Work out the finished part from the listing and answer in its coordinate system (mm). A direction names the side the tool comes from. Coordinates: 2 decimals unless noted, no trailing zeros. Order: outer loops, then holes, each group sorted by start corner. A loop starts at its lowest first (then second) coordinate and runs counter-clockwise, first axis right, second up.
1. Flat-ended cylindrical pins translate along their axes: pin 1 Ø6.5 at (x, z) = (6, 14) entering from +Y; pin 2 Ø6 at (x, y) = (-56.5, -6.5) entering from -Z; pin 3 Ø1.5 at (x, z) = (-53.5, -13.5) entering from -Y. Find the tip coordinate at first contact, or state that the pin passes through.
2. The part is cut by section A-A, the plane y = -9.75. Give the vertices of the cut face in (x, z).
3. The part is cut by section B-B, the plane x = -28. Give the vertices of the cut face in (y, z).
4. The part is cut by section C-C, the plane z = -0.5. Give the vertices of the cut face in (x, y).
5. A tool of negligible diameter and unlimited length cuts with its end or side. For faces 4 (the cylindrical face through (-72.49, -2.3, 19.54)), 5 (the flat face through (10, -2.5, -14)), 6 (the cylindrical face through (-35.5, 1.5, -9.23)), from which of +Z, -Z, +X, -X, +Y, -Y can it reach the whole face along a straight path? Write none if from no direction.
6. Determine the mould class of faces 1 (the flat face through (6, 0, 31)), 2 (the cylindrical face through (6, -8, 23)), 3 (the flat face through (6, 0, -31)) for opening direction Z: +Z half, -Z half, draft (parallel to the pull), parting line (faces both ways), or undercut.
7. Find the intervals of material crossed by probe 1 along Z at (x, y) = (6, -7.55); probe 2 along Z at (x, y) = (6, 8.4); probe 3 along Y at (x, z) = (7.75, -14), in increasing order.
```python
from build123d import *

# Parameters (mm, degrees)
PLATE_SKETCH_W               = 62
PLATE_SKETCH_H               = 23
PLATE_DEPTH                  = 12
TAPPED_HOLE_FACE_D           = 5
TAPPED_HOLE_FACE_CSINK_D     = 5.6
TAPPED_HOLE_FACE_CSINK_ANGLE = 90
RODS_DEPTH                   = 60
RODS_DEPTH_BACK              = 24
RODS_SKETCH_R                = 5
PISTON_SKETCH_R              = 6
PISTON_DEPTH                 = 1
TAPPED_HOLES_TOP_AT_2_COUNT  = 2
TAPPED_HOLES_TOP_AT_2_PITCH  = 50
SHCS_SEAT_SKETCH_R           = 5.5
SHCS_SEAT_DEPTH              = 6.5
SHCS_HEAD_SKETCH_R           = 5
SHCS_HEAD_DEPTH              = 6
SHCS_HEX_DEPTH               = 3
SHCS_CHAM_SIZE               = 0.6
SS_SEAT_SKETCH_R             = 4
SS_SEAT_DEPTH                = 2
SS_HEX_DEPTH                 = 4


with BuildPart() as part:
    # Plate_Sketch → Plate (new body)
    with BuildSketch(Plane(origin=(0, 0, 0), x_dir=(0, 0, -1), z_dir=(1, 0, 0))):
        Rectangle(PLATE_SKETCH_W, PLATE_SKETCH_H)
    extrude(amount=PLATE_DEPTH)

    # Tapped Hole Face (through all)
    with Locations(Plane(origin=(12, 0, 0), x_dir=(0, 0, -1), z_dir=(1, 0, 0))):
        with Locations((-25, 0), (25, 0)):
            CounterSinkHole(TAPPED_HOLE_FACE_D / 2, TAPPED_HOLE_FACE_CSINK_D / 2, counter_sink_angle=TAPPED_HOLE_FACE_CSINK_ANGLE)

    # Rods_Sketch → Rods (add, two sides: drawn at the far end of the back side and taken through both)
    with BuildSketch(Plane.ZY.offset(12).offset(-RODS_DEPTH_BACK)):
        with Locations((-14, 0)):
            Circle(RODS_SKETCH_R)
        with Locations(Location((14, 0, 0), (0, 0, 180))):
            Circle(RODS_SKETCH_R)
    extrude(amount=RODS_DEPTH + RODS_DEPTH_BACK)

    # Piston_Sketch → Piston (add)
    with BuildSketch(Plane.ZY.offset(72)):
        with Locations((-14, 0)):
            Circle(PISTON_SKETCH_R)
        with Locations((14, 0)):
            Circle(PISTON_SKETCH_R)
    extrude(amount=PISTON_DEPTH)

    # Tapped Holes Top Profile → Tapped Holes Top (revolve, cut)
    with BuildSketch(Plane(origin=(6, 11.5, -25), x_dir=(0, 0, 1), z_dir=(1, 0, 0))):
        Polygon((0, 0), (0, 6.499755867), (1.7, 6.2), (1.7, 6), (2, 6), (2, 0.3), (2.3, 0), align=None)
    tapped_holes_top = revolve(axis=Axis((6, 17.85, -25), (0, -1, 0)), mode=Mode.SUBTRACT)

    # Tapped Holes Top at 2: Tapped Holes Top ×2
    with Locations(*[(0, 0, i * TAPPED_HOLES_TOP_AT_2_PITCH) for i in range(1, TAPPED_HOLES_TOP_AT_2_COUNT)]):
        add(tapped_holes_top, mode=Mode.SUBTRACT)

    # Tapped Holes Top Mirror: Tapped Holes Top across plane
    add(tapped_holes_top.mirror(Plane.ZX), mode=Mode.SUBTRACT)

    # Tapped Holes Top Mirror copy 1 sketch → Tapped Holes Top Mirror copy 1 (revolve, cut)
    with BuildSketch(Plane(origin=(6, -11.5, 25), x_dir=(0, 0, 1), z_dir=(1, 0, 0))):
        Polygon((0, 0), (0, -6.499755867), (1.7, -6.2), (1.7, -6), (2, -6), (2, -0.3), (2.3, 0), align=None)
    revolve(axis=Axis((6, -17.85, 25), (0, -1, 0)), mode=Mode.SUBTRACT)

    # SHCS Seat_Sketch → SHCS Seat (cut)
    with BuildSketch(Plane(origin=(12, 0, 0), x_dir=(0, 0, -1), z_dir=(1, 0, 0))):
        with Locations((14, 0)):
            Circle(SHCS_SEAT_SKETCH_R)
    extrude(amount=-SHCS_SEAT_DEPTH, mode=Mode.SUBTRACT)

    # SHCS Head_Sketch → SHCS Head (add)
    with BuildSketch(Plane(origin=(5.5, 0, 0), x_dir=(0, 0, -1), z_dir=(1, 0, 0))):
        with Locations(Location((14, 0, 0), (0, 0, 180))):
            Circle(SHCS_HEAD_SKETCH_R)
    extrude(amount=SHCS_HEAD_DEPTH)

    # SHCS Hex_Sketch → SHCS Hex (cut)
    with BuildSketch(Plane(origin=(11.5, 0, 0), x_dir=(0, 0, -1), z_dir=(1, 0, 0))):
        Polygon((15.443375673, -2.5), (16.886751346, 0), (15.443375673, 2.5), (12.556624327, 2.5), (11.113248654, 0), (12.556624327, -2.5), align=None)
    extrude(amount=-SHCS_HEX_DEPTH, mode=Mode.SUBTRACT)

    # SHCS Cham
    shcs_cham_edges = [part.edges().sort_by_distance(p)[0] for p in [
        (11.5, 0, -19),
    ]]
    chamfer(shcs_cham_edges, length=SHCS_CHAM_SIZE)

    # SS Seat_Sketch → SS Seat (cut)
    with BuildSketch(Plane(origin=(0, 11.5, 0), x_dir=(-1, 0, 0), z_dir=(0, 1, 0))):
        with Locations(Location((-6, 14, 0), (0, 0, 90))):
            Circle(SS_SEAT_SKETCH_R)
    extrude(amount=-SS_SEAT_DEPTH, mode=Mode.SUBTRACT)

    # SS Hex_Sketch → SS Hex (cut)
    with BuildSketch(Plane(origin=(0, 9.5, 0), x_dir=(-1, 0, 0), z_dir=(0, 1, 0))):
        Polygon((-8, 12.845299462), (-6, 11.690598923), (-4, 12.845299462), (-4, 15.154700538), (-6, 16.309401077), (-8, 15.154700538), align=None)
    extrude(amount=-SS_HEX_DEPTH, mode=Mode.SUBTRACT)


solid = part.part
```
Geometry says:
1. pin 1: stops at y = 9.5
1. pin 2: stops at z = -17.57
1. pin 3: stops at y = -5
2. outline: (0, -31) - (12, -31) - (12, 31) - (0, 31) - close; hole circle Ø4 at (6, -25); hole circle Ø4 at (6, 25)
3. outline: circle Ø10 at (0, -14); circle Ø10 at (0, 14)
4. outline: (0, -11.5) - (12, -11.5) - (12, 11.5) - (0, 11.5) - close
5. face 4: -X
5. face 5: +X
5. face 6: none
6. face 1: +Z half
6. face 2: undercut
6. face 3: -Z half
7. probe 1: z = -31 to -27, -23 to 23, 27 to 31
7. probe 2: z = -31 to -27, -23 to 11.69, 16.31 to 23, 27 to 31
7. probe 3: y = -11.5 to -5.5, -5 to 5, 5.5 to 11.5
